```python
from build123d import *

# Parameters (mm, degrees)
SKETCH1_R           = 5
SKETCH1_R_2         = 1.5
SKETCH1_W           = 6
SKETCH1_H           = 6
BOSS_EXTRUDE1_DEPTH = 3
CUT_EXTRUDE1_DEPTH  = 51.318077676


with BuildPart() as part:
    # Sketch1 → Boss-Extrude1 (new body)
    with BuildSketch(Plane.XY):
        with BuildLine():
            Line((25.6, -12.03135802), (25.6, 8.75))
            ThreePointArc((25.6, 8.75), (24.135533906, 12.285533906), (20.6, 13.75))
            Line((20.6, 13.75), (-5, 13.75))
            ThreePointArc((-5, 13.75), (-8.535533906, 12.285533906), (-10, 8.75))
            Line((-10, 8.75), (-10, 0.66000458))
            Line((-10, 0.66000458), (-36.665975991, 10.365626108))
            ThreePointArc((-36.665975991, 10.365626108), (-43.074539812, 7.377263721), (-40.086177424, 0.9686999))
            Line((-40.086177424, 0.9686999), (31.330461755, -25.024830992))
            ThreePointArc((31.330461755, -25.024830992), (37.739025576, -22.036468605), (34.750663189, -15.627904785))
            Line((34.750663189, -15.627904785), (25.6, -12.29733576))
            Line((25.6, -12.29733576), (25.6, -12.03135802))
        make_face()
        Circle(SKETCH1_R, mode=Mode.SUBTRACT)
        with Locations((20.6, 8.75)):
            Circle(SKETCH1_R_2, mode=Mode.SUBTRACT)
        with Locations((20.6, -8.75)):
            Circle(SKETCH1_R_2, mode=Mode.SUBTRACT)
        with Locations((-38.376076708, 5.667163004)):
            Circle(SKETCH1_R_2, mode=Mode.SUBTRACT)
        with Locations((33.040562472, -20.326367889)):
            Circle(SKETCH1_R_2, mode=Mode.SUBTRACT)
        with Locations((12, 0)):
            Rectangle(SKETCH1_W, SKETCH1_H, mode=Mode.SUBTRACT)
    extrude(amount=BOSS_EXTRUDE1_DEPTH)

    # Sketch2 → Cut-Extrude1 (cut, through all)
    with BuildSketch(Plane(origin=(0, 0, 0), x_dir=(-1, 0, 0), z_dir=(0, 0, -1))):
        Polygon((24.449971921, 5.919364245), (27.269049783, 6.945424675), (28.9791505, 2.246961571), (26.160072638, 1.220901141), align=None)
        Polygon((-30.052200085, -13.917804068), (-27.233122222, -12.891743638), (-25.523021506, -17.590206742), (-28.342099368, -18.616267172), align=None)
    extrude(amount=-CUT_EXTRUDE1_DEPTH, mode=Mode.SUBTRACT)


solid = part.part
```
Can you work these out from the model? Positions are in its coordinate system, mm. A direction names the side the tool comes from. Give positions to 0.01 mm unless a question says otherwise; leave off trailing zeros. Loops run counter-clockwise (first coordinate to the right, second up) from the corner with the lowest first, then second, coordinate; pieces in that order, holes last. Notation, with made-up numbers: M 75.25,21 L 90.25,21 A20 cw 90.25,35 Z; hole C 32,31.25 d7. An arc over 180 degrees is marked long. One line per item, written item: value.
(1) Suppose I cut it at C-C on x = 0. List the corners of the cut face in (y, z) for me.
Returned:
outline: M -13.62,0 L -5,0 L -5,3 L -13.62,3 Z; M 5,0 L 13.75,0 L 13.75,3 L 5,3 Z
(2) Which directions (+Z, -Z, +X, -X, +Y, -Y) give clear straight access to the entire face, cutting with the end or side of a thin tool? Please do faces 1 (the face through (26.913, -18.096, 1.479)), 2 (the face through (6, -1, 0)), 3 (the face through (-25.317, 3.537, 1.479)).
Returned:
face 1: +Z, -Z
face 2: -Z, +X, -X, +Y, -Y
face 3: +Z, -Z, +Y
(3) I need wall thicknesses on line 1 (Y direction, x = 20.6, z = 2.05); line 2 (Y direction, x = -39, z = 2.35); line 3 (Y direction, x = -4.5, z = 0.45). Which ranges of each line are inside material? Lowest first, please.
Returned:
line 1: -21.12 to -10.25, -7.25 to 7.25, 10.25 to 13.75
line 2: 0.57 to 4.3, 7.03 to 10.63
line 3: -11.98 to -2.18, 2.18 to 13.75
(4) Suppose I cut it at A-A on y = -8.75. List the corners of the cut face in (x, z) for me, plus the area to 3 significant figures.
Returned:
outline: M -13.38,0 L 19.1,0 L 19.1,3 L -13.38,3 Z; M 22.1,0 L 25.6,0 L 25.6,3 L 22.1,3 Z
area: 108 mm^2
(5) Will these pins go through, and if not, where does the flat tip stop? pin 1 (1.5 mm diameter, centred on x = 13, z = 1, fed in from -Y); pin 2 (1.5 mm diameter, centred on y = -3, z = 1, fed in from +X).
Returned:
pin 1: y = -18.63
pin 2: x = 25.6
(6) Suppose I cut it at B-B on z = 1.05. List the corners of the cut face in (x, y) for me, plus the area to 3 significant figures.
Returned:
outline: M -40.09,0.97 L 31.33,-25.02 A5 ccw 34.75,-15.63 L 30.05,-13.92 L 28.34,-18.62 L 25.52,-17.59 L 27.23,-12.89 L 25.6,-12.3 L 25.6,8.75 A5 ccw 20.6,13.75 L -5,13.75 A5 ccw -10,8.75 L -10,0.66 L -24.45,5.92 L -26.16,1.22 L -28.98,2.25 L -27.27,6.95 L -36.67,10.37 A5 ccw Z; hole C -38.38,5.67 d3; hole C 0,0 d10; hole M 9,-3 L 15,-3 L 15,3 L 9,3 Z; hole C 20.6,-8.75 d3; hole C 20.6,8.75 d3; hole C 33.04,-20.33 d3
area: 1,350 mm^2
(7) We'd pull the mould along Y, two halves only. Please class faces 4 (the face through (-17.12, 3.25, 1.48)), 5 (the face through (-28.11, 4.63, 1.48)), 6 (the face through (-43.036, 7.48, 1.479)), 7 (the face through (6, -1, 3)): released by +Y, released by -Y, zero draft, split by the parting line, or undercut.
Returned:
face 4: released by +Y
face 5: undercut
face 6: split by the parting line
face 7: zero draft
